CAD build for the part. Positions are in the model's coordinates, mm. Coordinates: 2 decimals unless noted, no trailing zeros. Order: outer loops, then holes, each group sorted by start corner. A loop starts at its lowest first (then second) coordinate and runs counter-clockwise, first axis right, second up. Notation, with made-up numbers: M 77,-5.75 L 126,-5.75 A8 ccw 126,2.25 Z; hole C 75,71.25 d3. An arc over 180 degrees is marked long. One line per item, written item: value.
from build123d import *

# Parameters (mm, degrees)
BASE_W      = 80
BASE_H      = 50
BLOCK_DEPTH = 10
HOLES_2_R   = 3
HOLES_DEPTH = 49.218253805


with BuildPart() as part:
    # base → block (new body)
    with BuildSketch(Plane.XY):
        Rectangle(BASE_W, BASE_H)
    extrude(amount=BLOCK_DEPTH)

    # holes 2 → holes (cut, through all)
    with BuildSketch(Plane(origin=(0, 0, 10), x_dir=(-1, 0, 0), z_dir=(0, 0, -1))):
        with Locations((25, 15)):
            Circle(HOLES_2_R)
        with Locations((25, -15)):
            Circle(HOLES_2_R)
        with Locations((-25, 15)):
            Circle(HOLES_2_R)
        with Locations((-25, -15)):
            Circle(HOLES_2_R)
    extrude(amount=HOLES_DEPTH, mode=Mode.SUBTRACT)


solid = part.part
Q1. Drill centre lines: line 1 along X through (y, z) = (-15, 3.5); line 2 along Y through (x, z) = (-25, 7.75); line 3 along Y through (x, z) = (-23, 4). Where is each one in solid material? Low to high.
Recorded:
line 1: x = -40 to -28, -22 to 22, 28 to 40
line 2: y = -25 to -18, -12 to 12, 18 to 25
line 3: y = -25 to -17.24, -12.76 to 12.76, 17.24 to 25
Q2. Slice it at A-A (z = 1.5). List the corners of the cut face in (x, y), plus the area to 3 significant figures.
Recorded:
outline: M -40,-25 L 40,-25 L 40,25 L -40,25 Z; hole C -25,-15 d6; hole C -25,15 d6; hole C 25,-15 d6; hole C 25,15 d6
area: 3,890 mm^2
Q3. Slice it at C-C (x = -25). List the corners of the cut face in (y, z), plus the area to 3 significant figures.
Recorded:
outline: M -25,0 L -18,0 L -18,10 L -25,10 Z; M -12,0 L 12,0 L 12,10 L -12,10 Z; M 18,0 L 25,0 L 25,10 L 18,10 Z
area: 380 mm^2
Q4. Pin check, flat tip, straight feed: pin 1 Ø3.5 at (x, y) = (25, -15) entering from -Z. Stop position of the tip, or through.
Recorded:
pin 1: passes through
Q5. Mould opens along Y. For faces 1 (the face through (-1, 25, 5)), 2 (the face through (-1, 0, 0)), 3 (the face through (-24.35, 12.07, 5.07)) say: released by +Y, released by -Y, zero draft, split by the parting line, or undercut.
Recorded:
face 1: released by +Y
face 2: zero draft
face 3: undercut
Q6. Slice it at B-B (y = 15). List the corners of the cut face in (x, z).
Recorded:
outline: M -40,0 L -28,0 L -28,10 L -40,10 Z; M -22,0 L 22,0 L 22,10 L -22,10 Z; M 28,0 L 40,0 L 40,10 L 28,10 Z
